Answer from the drawing. Dimensions are ordinates in mm from the lowest x, y and z of the part. A direction names the side the tool comes from. Round coordinates to 2 decimals unless told otherwise and drop trailing zeros. Loops run counter-clockwise (first coordinate to the right, second up) from the corner with the lowest first, then second, coordinate; pieces in that order, holes last.
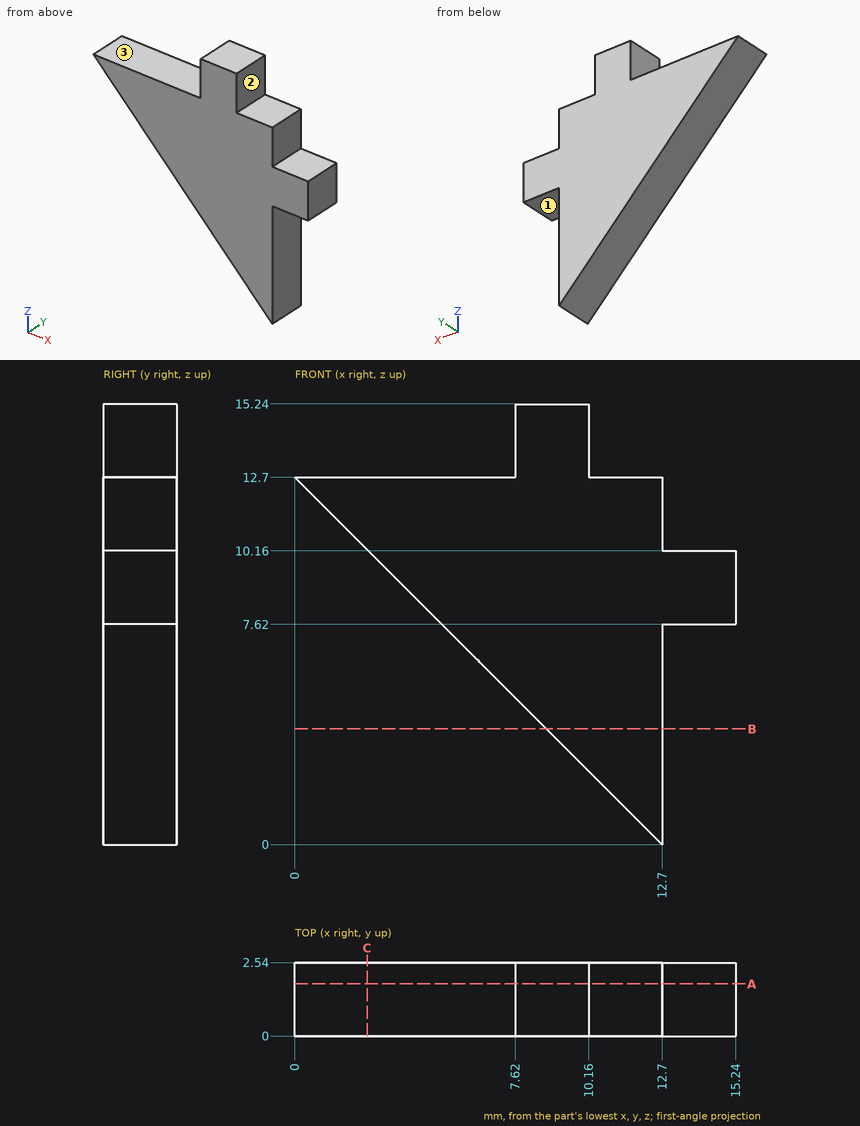
Item 1: Section A-A, the plane y = 1.8 is taken. Give the vertices of the cut face in (x, z), plus the area to 3 significant figures.
Item 2: For the marked faces 1, 2 and 3, determine the directions among +Z, -Z, +X, -X, +Y, -Y from which every point of the face is accessible in a straight line to the end or side of a thin tool.
Item 3: Straight lines are drawn through the part: line 1 (Z direction, x = 13.5, y = 1.7); line 2 (Z direction, x = 7.5, y = 2.1). For each, find the intervals that lie inside material, in ascending order.
Item 4: Section B-B, the plane z = 4 is taken. Give the vertices of the cut face in (x, y), plus the area to 3 significant figures.
Item 5: Section C-C, the plane x = 2.5 is taken. Give the vertices of the cut face in (y, z).
Item 6: Each of these flat-tipped pins is pushed along its axis until it touches: P1, Ø1, axis at x = 7.5, y = 1, coming from the -Z side; P2, Ø1.5, axis at y = 0.5, z = 2.5, coming from the -X side; P3, Ø1.3, axis at x = 14, y = 1.5, coming from the -Z side. Where does it stop, or does it pass through?
Answer below:
1. outline: (0, 12.7) - (12.7, 0) - (12.7, 7.62) - (15.24, 7.62) - (15.24, 10.16) - (12.7, 10.16) - (12.7, 12.7) - (10.16, 12.7) - (10.16, 15.24) - (7.62, 15.24) - (7.62, 12.7) - close
1. area: 93.5 mm2
2. face 1: -Z, +X, +Y, -Y
2. face 2: +Z, +X, +Y, -Y
2. face 3: +Z, -X, +Y, -Y
3. line 1: z = 7.62 to 10.16
3. line 2: z = 5.2 to 12.7
4. outline: (8.7, 0) - (12.7, 0) - (12.7, 2.54) - (8.7, 2.54) - close
4. area: 10.2 mm2
5. outline: (0, 10.2) - (2.54, 10.2) - (2.54, 12.7) - (0, 12.7) - close
6. P1: stops at z = 4.7
6. P2: stops at x = 9.45
6. P3: stops at z = 7.62
